from build123d import *

# Parameters (mm, degrees)
F0_R     = 15
F0_R_2   = 4.5
F1_DEPTH = 4
F2_R     = 12.75
F2_R_2   = 6
F3_DEPTH = 10
F4_R     = 2


with BuildPart() as f1:
    # F0 (on Top) → F1 (new body)
    with BuildSketch(Plane.XY):
        Circle(F0_R)
        Circle(F0_R_2, mode=Mode.SUBTRACT)
    extrude(amount=F1_DEPTH)

    # F2 (on face) → F3 (join)
    with BuildSketch(Plane(origin=(0, 0, 0), x_dir=(1, 0, 0), z_dir=(0, 0, -1))):
        Circle(F2_R)
        Circle(F2_R_2, mode=Mode.SUBTRACT)
    extrude(amount=F3_DEPTH)

    # F4
    f4_edges = [f1.edges().sort_by_distance(p)[0] for p in [
        (-15, 0, 4),
        (-4.5, 0, 4),
    ]]
    fillet(f4_edges, radius=F4_R)


solid = f1.part
For this review, take the finished solid that the model builds, in its own axes (mm). A direction names the side the tool comes from. Give positions to 0.01 mm unless a question says otherwise; leave off trailing zeros. Loops run counter-clockwise (first coordinate to the right, second up) from the corner with the lowest first, then second, coordinate; pieces in that order, holes last. Notation, with made-up numbers: M 27,67.25 L 67,67.25 A31 ccw 67,101.25 Z; hole C -31.5,12 d8. An arc over 180 degrees is marked long. Answer as a JSON object with one key per item and string values. Group by question number.
Q1. Add section A-A on y = 0. Give the boundary of the cut face in (x, z).
Q2. Add section C-C on z = -3.75. Give the boundary of the cut face in (x, y), and give its area (3 significant figures).
Q3. Insertion check: P1, Ø1, axis at y = -3.5, z = -8, coming from the -X side; P2, Ø8, axis at y = 5, z = -2.5, coming from the -X side; P3, Ø1.5, axis at x = -7, z = -0.5, coming from the -Y side. Each pin has a flat end and moves straight along its axis. Give the tip position at first contact, or say it passes through.
Q4. Tool access review of faces 1 (the cylindrical face through (-0.59, 4.46, 0.99)), 2 (the cylindrical face through (-6, 0, -5)): name each direction out of +Z, -Z, +X, -X, +Y, -Y from which nothing blocks a thin tool from reaching the whole face with its end or side.
Q5. For probe 1 along X at (y, z) = (0, -4.5); probe 2 along Y at (x, z) = (0, 0.7); probe 3 along X at (y, z) = (-1, -7.5), list the stretches that pass through material, from the lowest coordinate up. Write a range as [from, to].
Q6. Add section D-D on z = 1. Give the boundary of the cut face in (x, y), and give its area (3 significant figures).
Checked values:
{
 "1": {"outline": "M -15,0 L -12.75,0 L -12.75,-10 L -6,-10 L -6,0 L -4.5,0 L -4.5,2 A2 ccw -6.5,4 L -13,4 A2 ccw -15,2 Z; M 4.5,0 L 6,0 L 6,-10 L 12.75,-10 L 12.75,0 L 15,0 L 15,2 A2 ccw 13,4 L 6.5,4 A2 ccw 4.5,2 Z"},
 "2": {"outline": "C 0,0 d25.5; hole C 0,0 d12", "area": "398 mm²"},
 "3": {"P1": "x = -12.39", "P2": "x = -14.88", "P3": "y = -13.55"},
 "4": {"face 1": "+Z, -Z", "face 2": "-Z"},
 "5": {"probe 1": "[-12.75, -6], [6, 12.75]", "probe 2": "[-15, -4.5], [4.5, 15]", "probe 3": "[-12.71, -5.92], [5.92, 12.71]"},
 "6": {"outline": "C 0,0 d30; hole C 0,0 d9", "area": "643 mm²"}
}
